Design review of the part shown in the three views and the two pictorial views. Dimensions are in mm from the part's minimum x, y and z. Give positions to 0.01 mm unless a question says otherwise; leave off trailing zeros. Order: outer loops, then holes, each group sorted by start corner. A loop starts at its lowest first (then second) coordinate and runs counter-clockwise, first axis right, second up. Notation, with made-up numbers: (67, 46.25) -> (113, 46.25) arc R37 cw to (113, 82.25) -> close; hole circle Ø1 at (-35, -21.5). An arc over 180 degrees is marked (long way). Use one line per item in the form item = value.
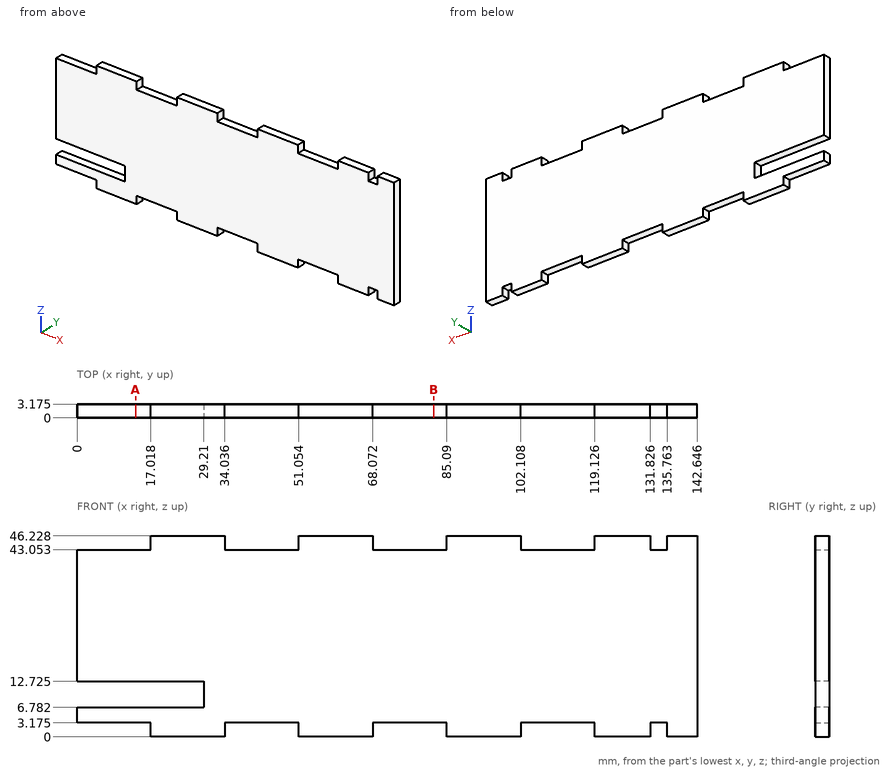
1. Add section B-B on x = 82. Give the boundary of the cut face in (y, z) (1 decimal).
Values:
outline = (0, 3.2) -> (3.2, 3.2) -> (3.2, 43.1) -> (0, 43.1) -> close
2. Add section A-A on x = 13.5. Give the boundary of the cut face in (y, z) (1 decimal), then the cut area to 3 significant figures.
Values:
outline = (0, 3.2) -> (3.2, 3.2) -> (3.2, 6.8) -> (0, 6.8) -> close; (0, 12.7) -> (3.2, 12.7) -> (3.2, 43.1) -> (0, 43.1) -> close
area = 108 mm^2
3. For L1, parallel to Z at x = 12, y = 3.05 (1 decimal); L2, parallel to Z at x = 20.5, y = 2.45 (1 decimal); L3, parallel to Z at x = 45.5, y = 2.5 (1 decimal), list the stretches that pass through material, from the lowest coordinate up.
Values:
L1 = 3.2 to 6.8, 12.7 to 43.1
L2 = 0 to 6.8, 12.7 to 46.2
L3 = 3.2 to 43.1
4. For pin 1 Ø1 at (x, y) = (42, 1.5) entering from +Z; pin 2 Ø1.6 at (y, z) = (2, 2) entering from -X; pin 3 Ø1.6 at (x, y) = (134, 1.5) entering from -Z (3 decimals), all flat-tipped, find the tip position at first contact; note any pin that passes through.
Values:
pin_1 = 43.05
pin_2 = 17.02
pin_3 = 3.175
